from build123d import *

# Parameters (mm, degrees)
F1_DEPTH = 1016


with BuildPart() as f1:
    # F0 (on Right) → F1 (new body)
    with BuildSketch(Plane.YZ):
        Polygon((-27.154803, 22.878646), (-7.154803, 22.878646), (-7.154803, 27.584923), (-9.154803, 29.584923), (-9.154803, 33.389069), (-25.154803, 33.389069), (-25.154803, 29.584923), (-27.154803, 27.584923), align=None)
        with BuildLine():
            ThreePointArc((-9.154803, 33.389069), (-8.569017, 34.803283), (-7.154803, 35.389069))
            Line((-7.154803, 35.389069), (-7.154803, 36.878646))
            ThreePointArc((-7.154803, 36.878646), (-8.569017, 37.464433), (-9.154803, 38.878646))
            Line((-9.154803, 38.878646), (-25.154803, 38.878646))
            ThreePointArc((-25.154803, 38.878646), (-25.74059, 37.464433), (-27.154803, 36.878646))
            Line((-27.154803, 36.878646), (-27.154803, 35.389069))
            ThreePointArc((-27.154803, 35.389069), (-25.74059, 34.803283), (-25.154803, 33.389069))
            Line((-25.154803, 33.389069), (-9.154803, 33.389069))
        make_face()
    extrude(amount=F1_DEPTH)


solid = f1.part
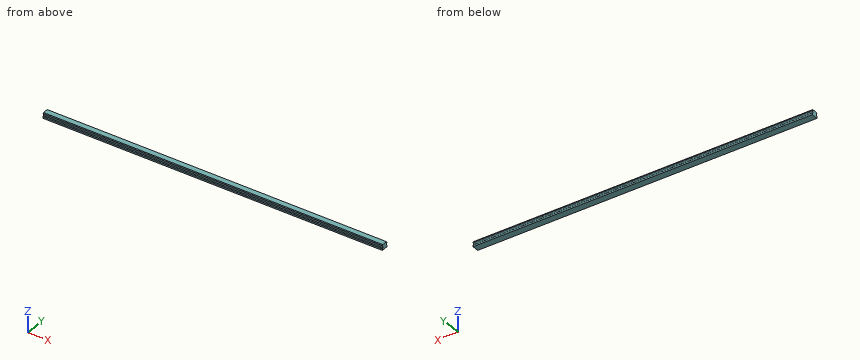
Read the model definition and answer for the solid it produces. Units are mm, in the model's axes. Round coordinates to 2 decimals unless told otherwise and drop trailing zeros. Write each loop counter-clockwise with the first axis right and the second up, starting at its lowest first coordinate (ties: lowest second). Pieces come first, ordered by that corner, then holes.
Q1. Straight lines are drawn through the part: line 1 (Z direction, x = 966.5, y = -8.5); line 2 (Y direction, x = 851.5, z = 38); line 3 (Y direction, x = 731, z = 34). For each, find the intervals that lie inside material, in ascending order.
Values:
line 1: z = 22.88 to 28.93, 34.87 to 37.4
line 2: y = -25.36 to -8.95
line 3: y = -25.25 to -9.06
Q2. Find section A-A on x = 913.5. Determine the outline of the cut face in (y, z), and give its area (3 significant figures).
Values:
outline: (-27.15, 22.88) - (-7.15, 22.88) - (-7.15, 27.58) - (-9.15, 29.58) - (-9.15, 33.39) arc R2 cw to (-7.15, 35.39) - (-7.15, 36.88) arc R2 cw to (-9.15, 38.88) - (-25.15, 38.88) arc R2 cw to (-27.15, 36.88) - (-27.15, 35.39) arc R2 cw to (-25.15, 33.39) - (-25.15, 29.58) - (-27.15, 27.58) - close
area: 288 mm2
Q3. Flat-ended cylindrical pins translate along their axes: P1, Ø1, axis at x = 270, z = 33.5, coming from the +Y side; P2, Ø4, axis at y = -17, z = 31.5, coming from the -X side; P3, Ø3, axis at x = 473.5, z = 31.5, coming from the -Y side. Find the tip coordinate at first contact, or state that the pin passes through.
Values:
P1: stops at y = -9.06
P2: stops at x = 0
P3: stops at y = -25.15
